from build123d import *

# Parameters (mm, degrees)
SKETCH1_W                    = 16.5
SKETCH1_H                    = 15
BASE_FLANGE1_DEPTH           = 3.175
EDGE_FLANGE1_STRIP_W         = 14.7
EDGE_FLANGE1_STRIP_H         = 3.175
EDGE_FLANGE1_STRIP_CUT_DEPTH = 15
EDGE_FLANGE1_DEPTH           = 15
SKETCH9_R                    = 4
CUT_EXTRUDE1_DEPTH           = 10
SKETCH10_R                   = 2
CUT_EXTRUDE2_DEPTH           = 10


# Sheet-metal steps are written as plain solids
with BuildPart() as part:
    # Sketch1 → Base-Flange1 (new body)
    with BuildSketch(Plane.XY):
        Rectangle(SKETCH1_W, SKETCH1_H)
    extrude(amount=BASE_FLANGE1_DEPTH)

    # Edge-Flange1 strip (across the edge) → Edge-Flange1 strip cut (cut)
    with BuildSketch(Plane(origin=(-8.25, 7.5, 3.175), x_dir=(1, 0, 0), z_dir=(0, -1, 0))):
        with Locations((-6.35, -1.5875)):
            Rectangle(EDGE_FLANGE1_STRIP_W, EDGE_FLANGE1_STRIP_H)
    extrude(amount=EDGE_FLANGE1_STRIP_CUT_DEPTH, mode=Mode.SUBTRACT)

    # Edge-Flange1 section (across the edge) → Edge-Flange1 (add)
    with BuildSketch(Plane(origin=(-8.25, 7.5, 3.175), x_dir=(1, 0, 0), z_dir=(0, -1, 0))):
        with BuildLine():
            Line((-3.175, 1), (-3.175, 10.825))
            Line((-3.175, 10.825), (0, 10.825))
            Line((0, 10.825), (0, 1))
            ThreePointArc((0, 1), (0.292893219, 0.292893219), (1, 0))
            Line((1, 0), (1, -3.175))
            ThreePointArc((1, -3.175), (-1.952170811, -1.952170811), (-3.175, 1))
        make_face()
    extrude(amount=EDGE_FLANGE1_DEPTH)

    # Sketch9 → Cut-Extrude1 (cut)
    with BuildSketch(Plane.XY.offset(3.175)):
        with Locations((0.63, 0)):
            Circle(SKETCH9_R)
    extrude(amount=-CUT_EXTRUDE1_DEPTH, mode=Mode.SUBTRACT)

    # Sketch10 → Cut-Extrude2 (cut)
    with BuildSketch(Plane(origin=(-8.25, 0, 0), x_dir=(0, 0, -1), z_dir=(1, 0, 0))):
        with Locations((-8.92, 0)):
            Circle(SKETCH10_R)
    extrude(amount=-CUT_EXTRUDE2_DEPTH, mode=Mode.SUBTRACT)


solid = part.part
Verification items for the finished model (mm, model axes). A direction names the side the tool comes from. Round coordinates to 2 decimals unless told otherwise and drop trailing zeros. Loops run counter-clockwise (first coordinate to the right, second up) from the corner with the lowest first, then second, coordinate; pieces in that order, holes last. Notation, with made-up numbers: (54.5, 21.25) - (100.5, 21.25) arc R25 cw to (100.5, 37.25) - close; hole circle Ø1 at (63.25, 80). An arc over 180 degrees is marked (long way). Answer in a Markdown table with one row per item. Add a question column.
Q1. Material ranges on line 1 (Z direction, x = 5.5, y = 7) (3 decimals); line 2 (X direction, y = -6.25, z = 12.25) (3 decimals); line 3 (Y direction, x = 0.63, z = 1.7), recorded low to high.
Q2. Tool access check on faces 1 (the face through (-8.25, 2, 10)), 2 (the face through (-9.815, -1.217, 10.507)). Record the directions out of +Z, -Z, +X, -X, +Y, -Y that give a thin tool (end or side, any length) a straight path to the whole face; none if there is none.
Q3. Section check C-C on x = 0.63. Enter the section's corners in (y, z) (3 decimals).
Q4. Section check B-B on z = 8.92. Enter the section's corners in (x, y) (3 decimals), plus the area to 3 significant figures.
Q5. Section check D-D on y = 2.75. Enter the section's corners in (x, z) (3 decimals), plus the area to 3 significant figures.
Q6. Section check A-A on y = 0. Enter the section's corners in (x, z) (3 decimals), plus the area to 3 significant figures.
Q7. Release check for a two-part mould opening along X. For faces 3 (the face through (-0.237, -3.905, 1.61)), 4 (the face through (8.25, 0, 2)), 5 (the face through (-4, 7.5, 3)) record: pulls with the +X half, pulls with the -X half, needs draft (parallel to the pull), parting line crosses it, or undercut.
Q8. Gauge pin test, flat end, axial feed: pin 1 (1 mm diameter, centred on y = 3.5, z = 9.5, fed in from +X). Record the tip position at first contact, or that the pin passes through.
Found:
| question | item | result |
|---|---|---|
| 1 | line 1 | z = 0 to 3.175 |
| 1 | line 2 | x = -11.425 to -8.25 |
| 1 | line 3 | y = -7.5 to -4, 4 to 7.5 |
| 2 | face 1 | +Z, +X, +Y, -Y |
| 2 | face 2 | +X, -X |
| 3 | outline | (-7.5, 0) - (-4, 0) - (-4, 3.175) - (-7.5, 3.175) - close; (4, 0) - (7.5, 0) - (7.5, 3.175) - (4, 3.175) - close |
| 4 | outline | (-11.425, -7.5) - (-8.25, -7.5) - (-8.25, -2) - (-11.425, -2) - close; (-11.425, 2) - (-8.25, 2) - (-8.25, 7.5) - (-11.425, 7.5) - close |
| 4 | area | 34.9 mm² |
| 5 | outline | (-11.425, 4.175) arc R4.175 ccw to (-7.25, 0) - (-2.275, 0) - (-2.275, 3.175) - (-7.25, 3.175) arc R1 cw to (-8.25, 4.175) - (-8.25, 14) - (-11.425, 14) - close; (3.535, 0) - (8.25, 0) - (8.25, 3.175) - (3.535, 3.175) - close |
| 5 | area | 74.9 mm² |
| 6 | outline | (-11.425, 4.175) arc R4.175 ccw to (-7.25, 0) - (-3.37, 0) - (-3.37, 3.175) - (-7.25, 3.175) arc R1 cw to (-8.25, 4.175) - (-8.25, 6.92) - (-11.425, 6.92) - close; (-11.425, 10.92) - (-8.25, 10.92) - (-8.25, 14) - (-11.425, 14) - close; (4.63, 0) - (8.25, 0) - (8.25, 3.175) - (4.63, 3.175) - close |
| 6 | area | 55.2 mm² |
| 7 | face 3 | undercut |
| 7 | face 4 | pulls with the +X half |
| 7 | face 5 | needs draft |
| 8 | pin 1 | stops at x = -8.25 |
